Model file for the job. Use its own axes, mm. A direction names the side the tool comes from. Coordinates: 2 decimals unless noted, no trailing zeros. Write each loop counter-clockwise with the first axis right and the second up, starting at its lowest first coordinate (ties: lowest second). Pieces come first, ordered by that corner, then holes. Notation, with made-up numbers: M 30,-6 L 70,-6 A32 ccw 70,20 Z; hole C 53.5,29.25 d11. An arc over 180 degrees is marked long. Put each result on its own line as item: value. Start each with the question number.
Q1. Cut at C-C (y = 4). Give the number of separate pieces and of enclosed holes in the cut face, then the cut area to 3 significant figures.
Q2. Cut at A-A (z = 0). Write the cut outline in (x, y).
Q3. Drop flat-ended pins along their axis: pin 1 (0.6 mm diameter, centred on y = 3.5, z = 4.5, fed in from +X); pin 2 (1.3 mm diameter, centred on y = 1.5, z = -7, fed in from -X); pin 3 (0.7 mm diameter, centred on y = 2.5, z = 8.5, fed in from -X); pin 4 (1 mm diameter, centred on y = 2, z = 4.5, fed in from -X). Give the stop position or say it passes through.
Q4. Which spindle directions (+Z, -Z, +X, -X, +Y, -Y) get a long thin tool onto all of the face, cutting with end or side? Do faces 1 (the flat face through (6.84, 2.5, 8.3)), 2 (the flat face through (13.76, 2.46, -9.4)), 3 (the flat face through (-15.251, 2, -7)), 4 (the flat face through (-14, 2, -7.869)). Say none if no direction does.
Q5. Cut at D-D (x = 13.5). Write the cut outline in (y, z).
Q6. Drill centre lines: line 1 along X through (y, z) = (4.25, -2.75); line 2 along X through (y, z) = (1.25, 0); line 3 along Z through (x, y) = (-10, 1.5). Where is each one in solid material? Low to high.
Q7. Pull direction Z, two halves, no side cores. Call faces 5 (the flat face through (-1.6, 2.5, -3.141)), 6 (the flat face through (14.175, 2, 0)), 7 (the flat face through (-10, 0, 0)): pulls with the +Z half, pulls with the -Z half, needs draft (parallel to the pull), parting line crosses it, or undercut.
Q8. Cut at B-B (x = -4). Write the cut outline in (y, z).
```python
from build123d import *

# Parameters (mm, degrees)
CROQUIS2_R                = 1.779687177
SALIENTE_EXTRUIR1_DEPTH   = 5
SALIENTE_EXTRUIR1_2_DEPTH = 5
SALIENTE_EXTRUIR1_3_DEPTH = 5
SALIENTE_EXTRUIR1_4_DEPTH = 5
SALIENTE_EXTRUIR1_5_DEPTH = 5
SALIENTE_EXTRUIR1_6_DEPTH = 5
SALIENTE_EXTRUIR1_7_DEPTH = 5
SALIENTE_EXTRUIR1_8_DEPTH = 5
SALIENTE_EXTRUIR1_9_DEPTH = 5
CROQUIS3_W                = 40.052022685
CROQUIS3_H                = 20
SALIENTE_EXTRUIR2_DEPTH   = 3
REDONDEO1_R               = 2


with BuildPart() as part:
    # Croquis2 → Saliente-Extruir1 (new body)
    with BuildSketch(Plane(origin=(0, 0, 0), x_dir=(1, 0, 0), z_dir=(0, 1, 0))):
        with Locations(Location((-10.039017014, 0, 0), (0, 0, 90))):
            Circle(CROQUIS2_R)
    extrude(amount=SALIENTE_EXTRUIR1_DEPTH)



with BuildPart() as body_2:
    # Croquis2 → Saliente-Extruir1 2 (new body)
    with BuildSketch(Plane(origin=(0, 0, 0), x_dir=(1, 0, 0), z_dir=(0, 1, 0))):
        with Locations(Location((9.986994329, 0, 0), (0, 0, 270))):
            Circle(CROQUIS2_R)
    extrude(amount=SALIENTE_EXTRUIR1_2_DEPTH)


with BuildPart() as body_3:
    # Croquis2 → Saliente-Extruir1 3 (new body)
    with BuildSketch(Plane(origin=(0, 0, 0), x_dir=(1, 0, 0), z_dir=(0, 1, 0))):
        Polygon((5.614984779, 10), (14.359003879, 10), (13.134466077, 8.775462198), (13.134466077, 7.868577354), (15.198808852, 7.868577354), (15.198808852, 6.711119422), (12.681851378, 4.194161948), (7.292137279, 4.194161948), (4.775179805, 6.711119422), (4.775179805, 7.868577354), (6.839522581, 7.868577354), (6.839522581, 8.775462198), align=None)
    extrude(amount=SALIENTE_EXTRUIR1_3_DEPTH)


with BuildPart() as body_4:
    # Croquis2 → Saliente-Extruir1 4 (new body)
    with BuildSketch(Plane(origin=(0, 0, 0), x_dir=(1, 0, 0), z_dir=(0, 1, 0))):
        Polygon((20, 4.155027818), (20, -4.155027818), (18.985761672, -3.14078949), (17.919495795, -3.14078949), (17.919495795, -5.172992947), (16.531532714, -5.172992947), (14.175115642, -2.816575874), (14.175115642, 2.816575874), (16.531532714, 5.172992947), (17.919495795, 5.172992947), (17.919495795, 3.14078949), (18.985761672, 3.14078949), align=None)
    extrude(amount=SALIENTE_EXTRUIR1_4_DEPTH)


with BuildPart() as body_5:
    # Croquis2 → Saliente-Extruir1 5 (new body)
    with BuildSketch(Plane(origin=(0, 0, 0), x_dir=(1, 0, 0), z_dir=(0, 1, 0))):
        Polygon((-0.026011343, 4.155027818), (-1.040249671, 3.14078949), (-2.106515548, 3.14078949), (-2.106515548, 5.172992947), (-3.494478629, 5.172992947), (-5.850895701, 2.816575874), (-5.850895701, -2.816575874), (-3.494478629, -5.172992947), (-2.106515548, -5.172992947), (-2.106515548, -3.14078949), (-1.040249671, -3.14078949), (-0.026011343, -4.155027818), (0.988226986, -3.14078949), (2.054492862, -3.14078949), (2.054492862, -5.172992947), (3.442455943, -5.172992947), (5.798873016, -2.816575874), (5.798873016, 2.816575874), (3.442455943, 5.172992947), (2.054492862, 5.172992947), (2.054492862, 3.14078949), (0.988226986, 3.14078949), align=None)
    extrude(amount=SALIENTE_EXTRUIR1_5_DEPTH)


with BuildPart() as body_6:
    # Croquis2 → Saliente-Extruir1 6 (new body)
    with BuildSketch(Plane(origin=(0, 0, 0), x_dir=(1, 0, 0), z_dir=(0, 1, 0))):
        Polygon((4.775179805, -6.711119422), (7.292137279, -4.194161948), (12.681851378, -4.194161948), (15.198808852, -6.711119422), (15.198808852, -7.868577354), (13.134466077, -7.868577354), (13.134466077, -8.775462198), (14.359003879, -10), (5.614984779, -10), (6.839522581, -8.775462198), (6.839522581, -7.868577354), (4.775179805, -7.868577354), align=None)
    extrude(amount=SALIENTE_EXTRUIR1_6_DEPTH)


with BuildPart() as body_7:
    # Croquis2 → Saliente-Extruir1 7 (new body)
    with BuildSketch(Plane(origin=(0, 0, 0), x_dir=(1, 0, 0), z_dir=(0, 1, 0))):
        Polygon((-12.733874064, -4.194161948), (-7.344159964, -4.194161948), (-4.82720249, -6.711119422), (-4.82720249, -7.868577354), (-6.891545266, -7.868577354), (-6.891545266, -8.775462198), (-5.667007464, -10), (-14.411026564, -10), (-13.186488762, -8.775462198), (-13.186488762, -7.868577354), (-15.250831538, -7.868577354), (-15.250831538, -6.711119422), align=None)
    extrude(amount=SALIENTE_EXTRUIR1_7_DEPTH)


with BuildPart() as body_8:
    # Croquis2 → Saliente-Extruir1 8 (new body)
    with BuildSketch(Plane(origin=(0, 0, 0), x_dir=(1, 0, 0), z_dir=(0, 1, 0))):
        Polygon((-16.583555399, -5.172992947), (-14.227138327, -2.816575874), (-14.227138327, 2.816575874), (-16.583555399, 5.172992947), (-17.97151848, 5.172992947), (-17.97151848, 3.14078949), (-19.037784357, 3.14078949), (-20.052022685, 4.155027818), (-20.052022685, -4.155027818), (-19.037784357, -3.14078949), (-17.97151848, -3.14078949), (-17.97151848, -5.172992947), align=None)
    extrude(amount=SALIENTE_EXTRUIR1_8_DEPTH)


with BuildPart() as body_9:
    # Croquis2 → Saliente-Extruir1 9 (new body)
    with BuildSketch(Plane(origin=(0, 0, 0), x_dir=(1, 0, 0), z_dir=(0, 1, 0))):
        Polygon((-5.667007464, 10), (-6.891545266, 8.775462198), (-6.891545266, 7.868577354), (-4.82720249, 7.868577354), (-4.82720249, 6.711119422), (-7.344159964, 4.194161948), (-12.733874064, 4.194161948), (-15.250831538, 6.711119422), (-15.250831538, 7.868577354), (-13.186488762, 7.868577354), (-13.186488762, 8.775462198), (-14.411026564, 10), align=None)
    extrude(amount=SALIENTE_EXTRUIR1_9_DEPTH)


with BuildPart() as part_1:
    add(part.part)

    add(body_2.part)  # Saliente-Extruir2 merges body 2

    add(body_3.part)  # Saliente-Extruir2 merges body 3

    add(body_4.part)  # Saliente-Extruir2 merges body 4

    add(body_5.part)  # Saliente-Extruir2 merges body 5

    add(body_6.part)  # Saliente-Extruir2 merges body 6

    add(body_7.part)  # Saliente-Extruir2 merges body 7

    add(body_8.part)  # Saliente-Extruir2 merges body 8

    add(body_9.part)  # Saliente-Extruir2 merges body 9
    # Croquis3 → Saliente-Extruir2 (add)
    with BuildSketch(Plane(origin=(0, 5, 0), x_dir=(1, 0, 0), z_dir=(0, 1, 0))):
        with Locations((-0.026011343, 0)):
            Rectangle(CROQUIS3_W, CROQUIS3_H)
    extrude(amount=SALIENTE_EXTRUIR2_DEPTH)

    # Redondeo1
    redondeo1_edges = [part_1.edges().sort_by_distance(p)[0] for p in [
        (-20.052022685, 8, 0),
        (-0.026011343, 8, 10),
        (20, 8, 0),
        (-0.026011343, 8, -10),
    ]]
    fillet(redondeo1_edges, radius=REDONDEO1_R)


solid = part_1.part
```
Computed values:
1. separate pieces: 9
1. enclosed holes: 0
1. area: 397 mm2
2. outline: M -20.05,0 L -14.23,0 L -14.23,5 L -11.82,5 L -11.82,0 L -8.26,0 L -8.26,5 L -5.85,5 L -5.85,0 L 5.8,0 L 5.8,5 L 8.21,5 L 8.21,0 L 11.77,0 L 11.77,5 L 14.18,5 L 14.18,0 L 20,0 L 20,6 A2 ccw 18,8 L -18.05,8 A2 ccw -20.05,6 Z
3. pin 1: x = 17.92
3. pin 2: x = -15.25
3. pin 3: x = -13.26
3. pin 4: x = -20.05
4. face 1: -Y
4. face 2: +X, -Y
4. face 3: -Z, -X, -Y
4. face 4: -X, -Y
5. outline: M 0,-10 L 6,-10 A2 ccw 8,-8 L 8,8 A2 ccw 6,10 L 0,10 L 0,9.14 L 5,9.14 L 5,7.87 L 0,7.87 L 0,5.01 L 5,5.01 L 5,-5.01 L 0,-5.01 L 0,-7.87 L 5,-7.87 L 5,-9.14 L 0,-9.14 Z
6. line 1: -20.05 to -14.23, -5.85 to 5.8, 14.18 to 20
6. line 2: -20.05 to -14.23, -11.82 to -8.26, -5.85 to 5.8, 8.21 to 11.77, 14.18 to 20
6. line 3: -10 to -4.19, -1.78 to 1.78, 4.19 to 10
7. face 5: pulls with the -Z half
7. face 6: undercut
7. face 7: needs draft
8. outline: M 0,-4.67 L 5,-4.67 L 5,-10 L 6,-10 A2 ccw 8,-8 L 8,8 A2 ccw 6,10 L 5,10 L 5,4.67 L 0,4.67 Z
